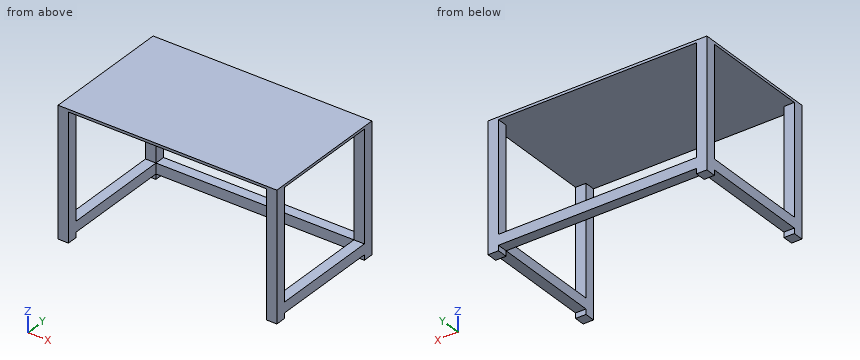
from build123d import *

# Parameters (mm, degrees)
F0_W     = 101.6
F0_H     = 101.6
F1_DEPTH = 1219.2
F2_W     = 2133.6
F2_H     = 1270
F3_DEPTH = 25.4
F4_W     = 101.6
F4_H     = 101.6
F5_DEPTH = 1066.8
F6_W     = 101.6
F6_H     = 101.6
F7_DEPTH = 1930.4


with BuildPart() as f1:
    # F0 (on Top) → F1 (new body)
    with BuildSketch(Plane.XY):
        with Locations((-1016, 584.2)):
            Rectangle(F0_W, F0_H)
        with Locations((-1016, -584.2)):
            Rectangle(F0_W, F0_H)
        with Locations((1016, -584.2)):
            Rectangle(F0_W, F0_H)
        with Locations((1016, 584.2)):
            Rectangle(F0_W, F0_H)
    extrude(amount=F1_DEPTH)

    # F2 (on face) → F3 (join)
    with BuildSketch(Plane.XY.offset(1219.2)):
        Rectangle(F2_W, F2_H)
    extrude(amount=F3_DEPTH)

    # F4 (on face) → F5 (join, through all)
    with BuildSketch(Plane.XZ.offset(-533.4)):
        with Locations((-1016, 101.6)):
            Rectangle(F4_W, F4_H)
        with Locations((1016, 101.6)):
            Rectangle(F4_W, F4_H)
    extrude(amount=F5_DEPTH)

    # F6 (on face) → F7 (join, through all)
    with BuildSketch(Plane(origin=(965.2, 0, 0), x_dir=(0, -1, 0), z_dir=(-1, 0, 0))):
        with Locations((-584.2, 101.6)):
            Rectangle(F6_W, F6_H)
    extrude(amount=F7_DEPTH)


solid = f1.part
The listing builds one solid part. Answer for the finished solid, in the listing's coordinates (mm). Give positions to 0.01 mm unless a question says otherwise; leave off trailing zeros. Loops run counter-clockwise (first coordinate to the right, second up) from the corner with the lowest first, then second, coordinate; pieces in that order, holes last. Notation, with made-up numbers: M 63.5,34 L 98.5,34 A26 ccw 98.5,51 Z; hole C -14,-3.5 d8. An arc over 180 degrees is marked long. Answer as CSV lines item,"result".
Item 1: The part is cut by section C-C (z = 632). Give the vertices of the cut face in (x, y).
Values follow:
outline,"M -1066.8,-635 L -965.2,-635 L -965.2,-533.4 L -1066.8,-533.4 Z; M -1066.8,533.4 L -965.2,533.4 L -965.2,635 L -1066.8,635 Z; M 965.2,-635 L 1066.8,-635 L 1066.8,-533.4 L 965.2,-533.4 Z; M 965.2,533.4 L 1066.8,533.4 L 1066.8,635 L 965.2,635 Z"
Item 2: The part is cut by section B-B (x = -79). Give the vertices of the cut face in (y, z), and give its area (3 significant figures).
Values follow:
outline,"M -635,1219.2 L 635,1219.2 L 635,1244.6 L -635,1244.6 Z; M 533.4,50.8 L 635,50.8 L 635,152.4 L 533.4,152.4 Z"
area,"42,600 mm^2"
Item 3: Given pin 1 Ø8 at (x, y) = (315, -479) entering from -Z, flat-ended and moving along its own axis, determine where the tip first touches the part or whether it passes through.
Values follow:
pin 1,"stops at z = 1219.2"
Item 4: Straight lines are drawn through the part: line 1 along Z through (x, y) = (-112.5, 564); line 2 along X through (y, z) = (-572.5, 288); line 3 along Z through (x, y) = (-918.5, 443.5). For each, find the intervals that lie inside material, in ascending order. Write a range as [from, to].
Values follow:
line 1,"z = [50.8, 152.4], [1219.2, 1244.6]"
line 2,"x = [-1066.8, -965.2], [965.2, 1066.8]"
line 3,"z = [1219.2, 1244.6]"
Item 5: The part is cut by section A-A (y = -59). Give the vertices of the cut face in (x, z), and give its area (3 significant figures).
Values follow:
outline,"M -1066.8,50.8 L -965.2,50.8 L -965.2,152.4 L -1066.8,152.4 Z; M -1066.8,1219.2 L 1066.8,1219.2 L 1066.8,1244.6 L -1066.8,1244.6 Z; M 965.2,50.8 L 1066.8,50.8 L 1066.8,152.4 L 965.2,152.4 Z"
area,"74,800 mm^2"
